```python
from build123d import *

# Parameters (mm, degrees)
BOSS_EXTRUDE1_DEPTH = 3
SKETCH2_W           = 10
SKETCH2_H           = 3
BOSS_EXTRUDE2_DEPTH = 3
SKETCH3_W           = 3
SKETCH3_H           = 13
BOSS_EXTRUDE3_DEPTH = 3
BOSS_EXTRUDE4_DEPTH = 15
FILLET1_R           = 3
FILLET2_R           = 2
CHAMFER1_SIZE       = 12
CHAMFER1_SIZE2      = 6.651708617
FILLET3_R           = 2
CHAMFER2_SIZE       = 12
CHAMFER2_SIZE2      = 6.651708617
FILLET4_R           = 2
FILLET5_R           = 5
FILLET7_R           = 2
BOSS_EXTRUDE5_DEPTH = 2


with BuildPart() as part:
    # Sketch1 → Boss-Extrude1 (new body)
    with BuildSketch(Plane.XY):
        Polygon((-10, 5), (-5, 5), (-5, 0), (0, 0), (0, 10), (-10, 10), align=None)
    extrude(amount=BOSS_EXTRUDE1_DEPTH)

    # Sketch2 → Boss-Extrude2 (add)
    with BuildSketch(Plane(origin=(0, 10, 0), x_dir=(1, 0, 0), z_dir=(0, 1, 0))):
        with Locations((-5, -1.5)):
            Rectangle(SKETCH2_W, SKETCH2_H)
    extrude(amount=BOSS_EXTRUDE2_DEPTH)

    # Sketch3 → Boss-Extrude3 (add)
    with BuildSketch(Plane(origin=(0, 0, 0), x_dir=(0, 0, -1), z_dir=(1, 0, 0))):
        with Locations((-1.5, 6.5)):
            Rectangle(SKETCH3_W, SKETCH3_H)
    extrude(amount=BOSS_EXTRUDE3_DEPTH)

    # Sketch4 → Boss-Extrude4 (add)
    with BuildSketch(Plane(origin=(0, 0, 0), x_dir=(-1, 0, 0), z_dir=(0, 0, -1))):
        Polygon((10, 13), (-3, 13), (-3, 9.459168036), (-3, 0), (0, 0), (0, 10), (10, 10), align=None)
    extrude(amount=BOSS_EXTRUDE4_DEPTH)

    # Fillet1
    fillet1_edges = [part.edges().sort_by_distance(p)[0] for p in [
        (-3.5, 13, 3),
        (3, 6.5, 3),
    ]]
    fillet(fillet1_edges, radius=FILLET1_R)

    # Fillet2
    fillet2_edges = [part.edges().sort_by_distance(p)[0] for p in [
        (-5, 5, 1.5),
        (-10, 5, 1.5),
        (-5, 0, 1.5),
    ]]
    fillet(fillet2_edges, radius=FILLET2_R)

    # Chamfer1
    chamfer1_edges = [part.edges().sort_by_distance(p)[0] for p in [
        (-10, 11.5, -15),
    ]]
    chamfer1_side = [part.faces().sort_by_distance(p)[0] for p in [
        (-10, 11.031627007, -5.158135036),
    ]]
    chamfer(chamfer1_edges, length=CHAMFER1_SIZE, length2=CHAMFER1_SIZE2, reference=chamfer1_side[0])

    # Fillet3
    fillet3_edges = [part.edges().sort_by_distance(p)[0] for p in [
        (-3.348291383, 11.5, -15),
        (-10, 11.5, -3),
    ]]
    fillet(fillet3_edges, radius=FILLET3_R)

    # Chamfer2
    chamfer2_edges = [part.edges().sort_by_distance(p)[0] for p in [
        (1.5, 0, -15),
    ]]
    chamfer2_side = [part.faces().sort_by_distance(p)[0] for p in [
        (1.031627007, 0, -5.158135036),
    ]]
    chamfer(chamfer2_edges, length=CHAMFER2_SIZE, length2=CHAMFER2_SIZE2, reference=chamfer2_side[0])

    # Fillet4
    fillet4_edges = [part.edges().sort_by_distance(p)[0] for p in [
        (1.5, 6.651708617, -15),
        (1.5, 0, -3),
    ]]
    fillet(fillet4_edges, radius=FILLET4_R)

    # Fillet5
    # the kernel refuses this fillet: 5 mm, written as the material it takes off along each edge
    with BuildSketch(Plane(origin=(-2, 8, 3), x_dir=(1, 0, 0), z_dir=(0, -1, 0))) as fillet5_piece_1:
        with BuildLine():
            CenterArc((2, -3), 3, 0, 90)
            Line((5, -3), (5, 0))
            Line((5, 0), (2, 0))
        make_face()
    revolve(axis=Axis((-2, 8, 3), (0, 0, 1)), revolution_arc=90, mode=Mode.SUBTRACT)
    with BuildSketch(Plane(origin=(3, 13, 3), x_dir=(0, -1, 0), z_dir=(0, 0, -1))) as fillet5_piece_2:
        with BuildLine():
            CenterArc((FILLET5_R, FILLET5_R), FILLET5_R, 180, 90)
            Line((0, FILLET5_R), (0, 0))
            Line((0, 0), (FILLET5_R, 0))
        make_face()
    extrude(amount=30.5, mode=Mode.SUBTRACT)

    # Fillet7
    fillet7_edges = [part.edges().sort_by_distance(p)[0] for p in [
        (-2.085100675, 13, -15),
        (-6.834340089, 13, -8.711001656),
        (-10, 13, -1.241382416),
        (-9.936295281, 13, -2.983524839),
        (-3.185278076, 13, -14.723258321),
        (3, 3.165659911, -8.711001656),
        (3, 0.063704719, -2.983524839),
        (3, 6.814721924, -14.723258321),
        (3, 7.914899325, -15),
        (1.535533906, 11.535533906, -15),
        (3, 0, -1.241382416),
        (2.121320344, 0, 2.121320344),
        (-10, 8.5, 3),
        (-10, 12.121320344, 2.121320344),
        (-5, 2.5, 3),
        (-7.5, 5, 3),
        (-1.5, 0, 3),
        (-4.414213562, 0.585786438, 3),
        (-9.414213562, 5.585786438, 3),
        (-5.585786438, 4.414213562, 3),
    ]]
    fillet(fillet7_edges, radius=FILLET7_R)

    # Sketch5 → Boss-Extrude5 (add)
    with BuildSketch(Plane(origin=(0, 0, 0), x_dir=(-1, 0, 0), z_dir=(0, 0, -1))):
        with BuildLine():
            Line((10, 8), (10, 7))
            ThreePointArc((10, 7), (9.414213562, 5.585786438), (8, 5))
            Line((8, 5), (7, 5))
            ThreePointArc((7, 5), (5.585786438, 4.414213562), (5, 3))
            Line((5, 3), (5, 2))
            ThreePointArc((5, 2), (4.414213562, 0.585786438), (3, 0))
            Line((3, 0), (2, 0))
            Line((2, 0), (2, 8))
            Line((2, 8), (10, 8))
        make_face()
    extrude(amount=BOSS_EXTRUDE5_DEPTH)


solid = part.part
```
Could you check a few things on this model? Use its own coordinates, in mm. A direction names the side the tool comes from. Round coordinates to 2 decimals unless told otherwise and drop trailing zeros. Loops run counter-clockwise (first coordinate to the right, second up) from the corner with the lowest first, then second, coordinate; pieces in that order, holes last. Notation, with made-up numbers: (39.25, -21.75) - (66.25, -21.75) arc R34 cw to (66.25, 17.25) - close; hole circle Ø6 at (-9, -2). An arc over 180 degrees is marked (long way). Use CSV: the item, a comma, the result in double quotes.
Item 1: If we mould it in two halves opening along X, with no side actions, what happens to faces 1 (the cylindrical face through (-3.198, 10.507, -14.716)), 2 (the flat face through (0.507, 3.206, -8.785)), 3 (the flat face through (-1.7, 7.2, 0))? For each: pulls with the +X half, pulls with the -X half, needs draft (parallel to the pull), parting line crosses it, or undercut.
Here are the results:
face 1,"pulls with the -X half"
face 2,"needs draft"
face 3,"undercut"
Item 2: If we section it at A-A on z = -1.75: List the corners of the cut face in (x, y) for me.
Here are the results:
outline,"(-10, 7) arc R2 ccw to (-8, 5) - (-7, 5) arc R2 cw to (-5, 3) - (-5, 2) arc R2 ccw to (-3, 0) - (-2, 0) - (-2, 8) - (-10, 8) - close; (-10, 10) - (0, 10) - (0, 0) - (1, 0) arc R2 ccw to (3, 2) - (3, 8) arc R5 ccw to (-2, 13) - (-8, 13) arc R2 ccw to (-10, 11) - close"
Item 3: Will these pins go through, and if not, where does the flat tip stop? pin 1 (3 mm diameter, centred on x = 1, y = 10.5, fed in from +Z); pin 2 (1.5 mm diameter, centred on x = -3.5, y = 7.5, fed in from -Z); pin 3 (0.5 mm diameter, centred on y = 2.5, z = 0, fed in from -X); pin 4 (3 mm diameter, centred on y = 6, z = -12.5, fed in from +X).
Here are the results:
pin 1,"stops at z = 2.97"
pin 2,"stops at z = -2"
pin 3,"stops at x = -5"
pin 4,"stops at x = 3"
Item 4: I need wall thicknesses on L1, parallel to Z at x = -7.25, y = 7.5; L2, parallel to X at y = 4, z = -4.75; L3, parallel to Y at x = -3.25, z = -9.5. Which ranges of each line are inside material? Lowest first, please. Write a range as [from, to].
Here are the results:
L1,"z = [-2, 3]"
L2,"x = [0, 3]"
L3,"y = [10, 13]"
Item 5: For faces 4 (the flat face through (-5, 2.5, -0.5)), 5 (the cylindrical face through (-5.04, 12.14, 2.1)), 6 (the cylindrical face through (-7.51, 5.57, 2.4)), which set-ups out of +Z, -Z, +X, -X, +Y, -Y let a thin tool reach every point of the face, with its end or its side?
Here are the results:
face 4,"+Z, -Z, -X, -Y"
face 5,"+Z, +X, -X, +Y"
face 6,"+Z, -X, -Y"
